from build123d import *

# Parameters (mm, degrees)
SKETCH_1_W          = 60
SKETCH_1_H          = 14.5
SKETCH_1_R          = 1.6
EXTRUDE_1_DEPTH     = 1
SKETCH_2_W          = 120.5
SKETCH_2_H          = 75
SKETCH_2_R          = 1.6
EXTRUDE_2_DEPTH     = 1
SKETCH_3_R          = 1.6
CUT_EXTRUDE_1_DEPTH = 10
SKETCH_4_W          = 30
SKETCH_4_H          = 75
EXTRUDE_3_DEPTH     = 1
FILLET_1_R          = 7
SKETCH_5_W          = 10
SKETCH_5_H          = 14.5
CUT_EXTRUDE_2_DEPTH = 10
FILLET_2_R          = 7
FILLET_3_R          = 2


with BuildPart() as part:
    # 草图1 → 凸台-拉伸1 (new body)
    with BuildSketch(Plane.XY):
        with Locations((0, -2.75)):
            Rectangle(SKETCH_1_W, SKETCH_1_H)
        with Locations((-10, 0)):
            Circle(SKETCH_1_R, mode=Mode.SUBTRACT)
        with Locations((10, 0)):
            Circle(SKETCH_1_R, mode=Mode.SUBTRACT)
    extrude(amount=EXTRUDE_1_DEPTH)

    # 草图2 → 凸台-拉伸2 (add)
    with BuildSketch(Plane(origin=(0, 0, 0), x_dir=(-1, 0, 0), z_dir=(0, 0, -1))):
        with Locations((-22.5, 42)):
            Rectangle(SKETCH_2_W, SKETCH_2_H)
        with Locations((-76.75, 52)):
            Circle(SKETCH_2_R, mode=Mode.SUBTRACT)
        with Locations((-76.75, 32)):
            Circle(SKETCH_2_R, mode=Mode.SUBTRACT)
    extrude(amount=-EXTRUDE_2_DEPTH)

    # 草图3 → 切除-拉伸1 (cut)
    with BuildSketch(Plane(origin=(0, 0, 0), x_dir=(-1, 0, 0), z_dir=(0, 0, -1))):
        with Locations((-27.5, 75.5)):
            Circle(SKETCH_3_R)
        with Locations((-7.5, 75.5)):
            Circle(SKETCH_3_R)
    extrude(amount=-CUT_EXTRUDE_1_DEPTH, mode=Mode.SUBTRACT)

    # 草图4 → 凸台-拉伸3 (add)
    with BuildSketch(Plane(origin=(0, 0, 0), x_dir=(-1, 0, 0), z_dir=(0, 0, -1))):
        with Locations((52.75, 42)):
            Rectangle(SKETCH_4_W, SKETCH_4_H)
    extrude(amount=-EXTRUDE_3_DEPTH)

    # 圆角1
    fillet_1_edges = [part.edges().sort_by_distance(p)[0] for p in [
        (30, -10, 0.5),
        (30, 4.5, 0.5),
    ]]
    fillet(fillet_1_edges, radius=FILLET_1_R)

    # 草图5 → 切除-拉伸2 (cut)
    with BuildSketch(Plane(origin=(0, 0, 0), x_dir=(-1, 0, 0), z_dir=(0, 0, -1))):
        with Locations((25, -2.75)):
            Rectangle(SKETCH_5_W, SKETCH_5_H)
    extrude(amount=-CUT_EXTRUDE_2_DEPTH, mode=Mode.SUBTRACT)

    # 圆角2
    fillet_2_edges = [part.edges().sort_by_distance(p)[0] for p in [
        (-20, -10, 0.5),
        (-20, 4.5, 0.5),
    ]]
    fillet(fillet_2_edges, radius=FILLET_2_R)

    # 圆角3
    fillet_3_edges = [part.edges().sort_by_distance(p)[0] for p in [
        (82.75, 4.5, 0.5),
        (82.75, 79.5, 0.5),
        (-67.75, 79.5, 0.5),
        (-67.75, 4.5, 0.5),
    ]]
    fillet(fillet_3_edges, radius=FILLET_3_R)


solid = part.part
Geometry check sheet. Reference: the model listing, model coordinates, mm. Round coordinates to 2 decimals unless told otherwise and drop trailing zeros. Write each loop counter-clockwise with the first axis right and the second up, starting at its lowest first coordinate (ties: lowest second). Pieces come first, ordered by that corner, then holes.
Item 1: Go/stop test with a flat-tipped pin: pin 1 Ø2.5 at (x, y) = (76.75, 32) entering from -Z. Record where the tip stops, or that it passes through.
Determined:
pin 1: passes through
Item 2: Section check B-B (y = 52). Record the boundary of the cut face in (x, z), plus the area to 3 significant figures.
Determined:
outline: (-67.75, 0) - (75.15, 0) - (75.15, 1) - (-67.75, 1) - close; (78.35, 0) - (82.75, 0) - (82.75, 1) - (78.35, 1) - close
area: 147 mm2
Item 3: Section check C-C (z = 0.25). Record the boundary of the cut face in (x, y), plus the area to 3 significant figures.
Determined:
outline: (-67.75, 6.5) arc R2 ccw to (-65.75, 4.5) - (-27, 4.5) arc R7 cw to (-20, -2.5) - (-20, -3) arc R7 ccw to (-13, -10) - (23, -10) arc R7 ccw to (30, -3) - (30, -2.5) arc R7 cw to (37, 4.5) - (80.75, 4.5) arc R2 ccw to (82.75, 6.5) - (82.75, 77.5) arc R2 ccw to (80.75, 79.5) - (-65.75, 79.5) arc R2 ccw to (-67.75, 77.5) - close; hole circle Ø3.2 at (-10, 0); hole circle Ø3.2 at (7.5, 75.5); hole circle Ø3.2 at (10, 0); hole circle Ø3.2 at (27.5, 75.5); hole circle Ø3.2 at (76.75, 32); hole circle Ø3.2 at (76.75, 52)
area: 12,000 mm2
Item 4: Section check A-A (x = 76.75). Record the boundary of the cut face in (y, z).
Determined:
outline: (4.5, 0) - (30.4, 0) - (30.4, 1) - (4.5, 1) - close; (33.6, 0) - (50.4, 0) - (50.4, 1) - (33.6, 1) - close; (53.6, 0) - (79.5, 0) - (79.5, 1) - (53.6, 1) - close
Item 5: Mould release check, pull along Y, two halves, no side actions. Record for faces 1 (the face through (-18, -7.9, 0.5)), 2 (the face through (9, 35, 1)), 3 (the face through (75.224, 52.481, 0.493)): +Y half, -Y half, draft (parallel to the pull), parting line (faces both ways), or undercut.
Determined:
face 1: -Y half
face 2: draft
face 3: undercut
Item 6: Section check D-D (x = -10). Record the boundary of the cut face in (y, z), plus the area to 3 significant figures.
Determined:
outline: (-10, 0) - (-1.6, 0) - (-1.6, 1) - (-10, 1) - close; (1.6, 0) - (79.5, 0) - (79.5, 1) - (1.6, 1) - close
area: 86.3 mm2
Item 7: Material ranges on line 1 along Y through (x, z) = (76.75, 0.3); line 2 along X through (y, z) = (75.5, 0.55); line 3 along Y through (x, z) = (10, 0.35), recorded low to high.
Determined:
line 1: y = 4.5 to 30.4, 33.6 to 50.4, 53.6 to 79.5
line 2: x = -67.75 to 5.9, 9.1 to 25.9, 29.1 to 82.75
line 3: y = -10 to -1.6, 1.6 to 79.5
